Build history of the part. All positions in model axes, mm. Face numbers are marked on the shaded views. Round coordinates to 2 decimals unless told otherwise and drop trailing zeros. Write each loop counter-clockwise with the first axis right and the second up, starting at its lowest first coordinate (ties: lowest second). Pieces come first, ordered by that corner, then holes. Notation, with made-up numbers: M 24,57 L 30,57 A17 cw 30,87 Z; hole C 8,9.25 d1. An arc over 180 degrees is marked long. Use a Markdown table: item, result.
from build123d import *

# Parameters (mm, degrees)
SKETCH1_W               = 200
SKETCH1_H               = 856
BASE_FLANGE1_DEPTH      = 2
EDGE_FLANGE1_DEPTH      = 856
EDGE_FLANGE1_BEND_DEPTH = 856


# Sheet-metal steps are written as plain solids
with BuildPart() as part:
    # Sketch1 → Base-Flange1 (new body)
    with BuildSketch(Plane(origin=(0, 0, 0), x_dir=(1, 0, 0), z_dir=(0, 1, 0))):
        Rectangle(SKETCH1_W, SKETCH1_H)
    extrude(amount=-BASE_FLANGE1_DEPTH)

    # Edge-Flange1 section (across the edge) → Edge-Flange1 (add)
    with BuildSketch(Plane(origin=(103, 0, 428), x_dir=(-1, 0, 0), z_dir=(0, 0, -1))):
        with BuildLine():
            Line((-2, 3), (-2, 20))
            Line((-2, 20), (0, 20))
            Line((0, 20), (0, 3))
            ThreePointArc((0, 3), (0.878679656, 0.878679656), (3, 0))
            Line((3, 0), (3, -2))
            ThreePointArc((3, -2), (-0.535533906, -0.535533906), (-2, 3))
        make_face()
    extrude(amount=EDGE_FLANGE1_DEPTH)

    # Edge-Flange1 section 2 (across the edge) → Edge-Flange1 bend (add)
    with BuildSketch(Plane(origin=(-103, 0, -428), x_dir=(1, 0, 0), z_dir=(0, 0, 1))):
        with BuildLine():
            Line((-2, 3), (-2, 20))
            Line((-2, 20), (0, 20))
            Line((0, 20), (0, 3))
            ThreePointArc((0, 3), (0.878679656, 0.878679656), (3, 0))
            Line((3, 0), (3, -2))
            ThreePointArc((3, -2), (-0.535533906, -0.535533906), (-2, 3))
        make_face()
    extrude(amount=EDGE_FLANGE1_BEND_DEPTH)


solid = part.part
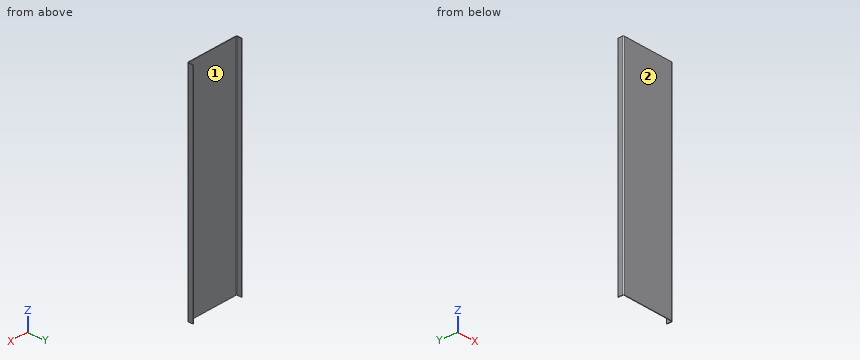
Q1. Two-plate mould, pull along X, no slides. Class the marked faces 1 and 2: +X half, -X half, draft (parallel to the pull), parting line (faces both ways), or undercut.
Response values:
| item | result |
|---|---|
| face 1 | undercut |
| face 2 | draft |
Q2. Cut at B-B on z = 72.5. Give the cut face in (x, y), and give its area (3 significant figures).
Response values:
| item | result |
|---|---|
| outline | M -105,3 A5 ccw -100,-2 L 100,-2 A5 ccw 105,3 L 105,20 L 103,20 L 103,3 A3 cw 100,0 L -100,0 A3 cw -103,3 L -103,20 L -105,20 Z |
| area | 493 mm2 |
Q3. Cut at A-A on y = 10. Give the cut face in (x, z).
Response values:
| item | result |
|---|---|
| outline | M -105,-428 L -103,-428 L -103,428 L -105,428 Z; M 103,-428 L 105,-428 L 105,428 L 103,428 Z |
Q4. Drill centre lines: L1, parallel to X at y = 11, z = 17; L2, parallel to Y at x = 49, z = 49.5. Where is each one in solid material? Low to high.
Response values:
| item | result |
|---|---|
| L1 | x = -105 to -103, 103 to 105 |
| L2 | y = -2 to 0 |
Q5. Cut at C-C on x = -31. Give the cut face in (y, z), and give its area (3 significant figures).
Response values:
| item | result |
|---|---|
| outline | M -2,-428 L 0,-428 L 0,428 L -2,428 Z |
| area | 1,710 mm2 |
